Build history of the part. All positions in model axes, mm. Face numbers are marked on the shaded views. A direction names the side the tool comes from. Round coordinates to 2 decimals unless told otherwise and drop trailing zeros. Loops run counter-clockwise (first coordinate to the right, second up) from the corner with the lowest first, then second, coordinate; pieces in that order, holes last. Notation, with made-up numbers: (-19.5, -28.75) - (1.5, -28.75) arc R19 ccw to (1.5, -23.75) - close; hole circle Ø5 at (-1.5, 28). An arc over 180 degrees is marked (long way). Use one line per item in the form item = value. Start each with the question number.
Q1. Pin check, flat tips, straight feed: pin 1 (1 mm diameter, centred on x = -56.5, y = 11, fed in from -Z); pin 2 (5 mm diameter, centred on x = -8, z = -5.5, fed in from +Y); pin 3 (1.5 mm diameter, centred on x = -13, z = -4.5, fed in from -Y); pin 4 (1 mm diameter, centred on x = 57, y = 11.5, fed in from +Z). Stop position of each tip, or through.
Q2. Drill centre lines: line 1 (Z direction, x = -25, y = 8.25); line 2 (X direction, y = 3.5, z = -2); line 3 (Y direction, x = -15, z = 6.75). Where is each one in solid material? Low to high.
Q3. 3-axis set-ups, long thin cutter, end or side, ignore diameter. For the marked faces 5 and 6: which of +Z, -Z, +X, -X, +Y, -Y reach the whole face in a straight line?
Q4. Saw through at A-A (x = -44.5). Give the cut face in (y, z), then the cut area to 3 significant figures.
Q5. Mould opens along X. For the marked faces 1, 2, 3 and 4 say: released by +X, released by -X, zero draft, split by the parting line, or undercut.
Q6. Saw through at C-C (z = -1.75). Give the cut face in (x, y), then the cut area to 3 significant figures.
Q7. Saw through at B-B (y = 4.75). Give the cut face in (x, z).
Q8. Saw through at D-D (z = 6.5). Give the cut face in (x, y), then the cut area to 3 significant figures.
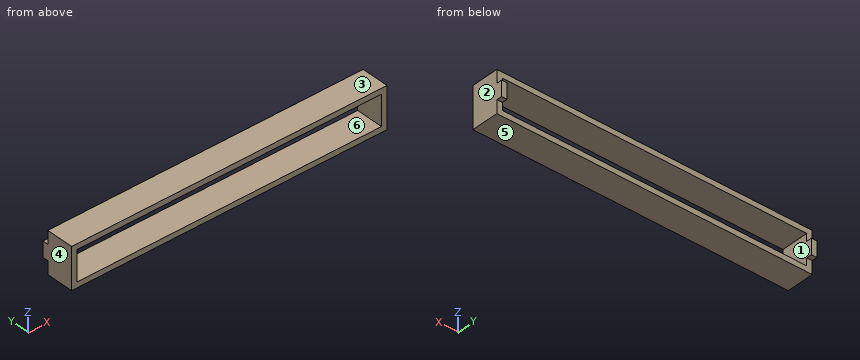
```python
from build123d import *

# Parameters (mm, degrees)
SKETCH1_W           = 115
SKETCH1_H           = 15
SKETCH1_W_2         = 111
SKETCH1_H_2         = 11
BOSS_EXTRUDE1_DEPTH = 10
SKETCH2_W           = 2
SKETCH2_H           = 5.6
BOSS_EXTRUDE2_DEPTH = 2


with BuildPart() as part:
    # Sketch1 → Boss-Extrude1 (new body)
    with BuildSketch(Plane(origin=(0, 0, 0), x_dir=(1, 0, 0), z_dir=(0, 1, 0))):
        Rectangle(SKETCH1_W, SKETCH1_H)
        Rectangle(SKETCH1_W_2, SKETCH1_H_2, mode=Mode.SUBTRACT)
    extrude(amount=BOSS_EXTRUDE1_DEPTH)

    # Sketch2 → Boss-Extrude2 (add)
    with BuildSketch(Plane(origin=(0, 10, 0), x_dir=(1, 0, 0), z_dir=(0, 1, 0))):
        with Locations((-56.5, 0)):
            Rectangle(SKETCH2_W, SKETCH2_H)
        with Locations((56.5, 0)):
            Rectangle(SKETCH2_W, SKETCH2_H)
    extrude(amount=BOSS_EXTRUDE2_DEPTH)


solid = part.part
```
Report:
q1.pin_1 = -2.8
q1.pin_2 = 10
q1.pin_3 = through
q1.pin_4 = 2.8
q2.line_1 = -7.5 to -5.5, 5.5 to 7.5
q2.line_2 = -57.5 to -55.5, 55.5 to 57.5
q2.line_3 = 0 to 10
q3.face_5 = -Z, +X, -X, +Y, -Y
q3.face_6 = +Y, -Y
q4.outline = (0, -7.5) - (10, -7.5) - (10, -5.5) - (0, -5.5) - close; (0, 5.5) - (10, 5.5) - (10, 7.5) - (0, 7.5) - close
q4.area = 40.0 mm²
q5.face_1 = undercut
q5.face_2 = released by +X
q5.face_3 = zero draft
q5.face_4 = released by -X
q6.outline = (-57.5, 0) - (-55.5, 0) - (-55.5, 12) - (-57.5, 12) - close; (55.5, 0) - (57.5, 0) - (57.5, 12) - (55.5, 12) - close
q6.area = 48.0 mm²
q7.outline = (-57.5, -7.5) - (57.5, -7.5) - (57.5, 7.5) - (-57.5, 7.5) - close; hole (-55.5, -5.5) - (55.5, -5.5) - (55.5, 5.5) - (-55.5, 5.5) - close
q8.outline = (-57.5, 0) - (57.5, 0) - (57.5, 10) - (-57.5, 10) - close
q8.area = 1,150 mm²
